Check sheet for the drawn part. Datum: minimum x, y, z corner. Units: mm. Round coordinates to 2 decimals unless told otherwise and drop trailing zeros. Order: outer loops, then holes, each group sorted by start corner. A loop starts at its lowest first (then second) coordinate and runs counter-clockwise, first axis right, second up.
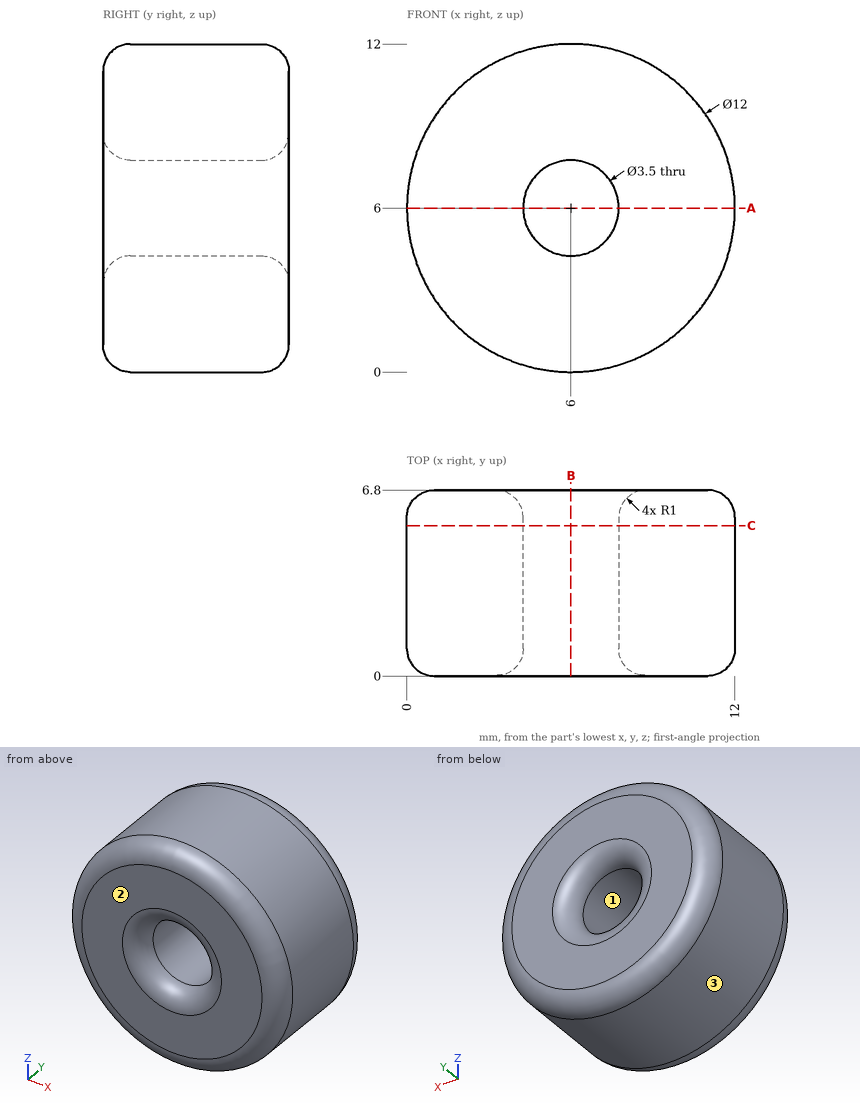
(1) Draft check along X on the marked faces 1, 2 and 3. Enter one of: released by +X, released by -X, zero draft, split by the parting line, or undercut.
Returned:
face 1: undercut
face 2: zero draft
face 3: split by the parting line
(2) Sectioned sample at B-B, the plane x = 6. Record the cut outline in (y, z).
Returned:
outline: (0, 1) arc R1 ccw to (1, 0) - (5.8, 0) arc R1 ccw to (6.8, 1) - (6.8, 3.25) arc R1 ccw to (5.8, 4.25) - (1, 4.25) arc R1 ccw to (0, 3.25) - close; (0, 8.75) arc R1 ccw to (1, 7.75) - (5.8, 7.75) arc R1 ccw to (6.8, 8.75) - (6.8, 11) arc R1 ccw to (5.8, 12) - (1, 12) arc R1 ccw to (0, 11) - close
(3) Material ranges on line 1 (Z direction, x = 6, y = 5); line 2 (Y direction, x = 3.25, z = 1.75); line 3 (Z direction, x = 3, y = 5.5), recorded low to high.
Returned:
line 1: z = 0 to 4.25, 7.75 to 12
line 2: y = 0 to 6.8
line 3: z = 0.8 to 11.2
(4) Sectioned sample at C-C, the plane y = 5.5. Record the cut outline in (x, z), and give its area (3 significant figures).
Returned:
outline: circle Ø12 at (6, 6); hole circle Ø3.5 at (6, 6)
area: 103 mm2
(5) Depth check by flat-ended pin: P1, Ø4, axis at y = 4, z = 2.5, coming from the +X side; P2, Ø2, axis at y = 6, z = 9.5, coming from the +X side; P3, Ø3, axis at x = 5.5, y = 3, coming from the -Z side. Enter the tip coordinate at first touch or a pass-through.
Returned:
P1: stops at x = 11.81
P2: stops at x = 11.45
P3: stops at z = 0
(6) Sectioned sample at A-A, the plane z = 6. Record the cut outline in (x, y).
Returned:
outline: (0, 1) arc R1 ccw to (1, 0) - (3.25, 0) arc R1 ccw to (4.25, 1) - (4.25, 5.8) arc R1 ccw to (3.25, 6.8) - (1, 6.8) arc R1 ccw to (0, 5.8) - close; (7.75, 1) arc R1 ccw to (8.75, 0) - (11, 0) arc R1 ccw to (12, 1) - (12, 5.8) arc R1 ccw to (11, 6.8) - (8.75, 6.8) arc R1 ccw to (7.75, 5.8) - close
